Model file for the job. Use its own axes, mm. Face numbers are marked on the shaded views. Round coordinates to 2 decimals unless told otherwise and drop trailing zeros. Loops run counter-clockwise (first coordinate to the right, second up) from the corner with the lowest first, then second, coordinate; pieces in that order, holes last. Notation, with made-up numbers: M 41.5,39 L 57.5,39 A16 ccw 57.5,55 Z; hole C 89,83.5 d2. An arc over 180 degrees is marked long. Use a Markdown table: item, result. Add a question column.
Item 1: Saw through at C-C on x = -58. Write the cut outline in (y, z), then the cut area to 3 significant figures.
Item 2: Saw through at B-B on x = -4. Give the number of separate pieces and of enclosed holes in the cut face, then the cut area to 3 significant figures.
Item 3: Saw through at A-A on y = -32. Write the cut outline in (x, z), then the cut area to 3 significant figures.
Item 4: Pin check, flat tips, straight feed: P1, Ø8, axis at x = 56.5, y = 47, coming from the +Z side; P2, Ø3, axis at x = -75, z = 8.5, coming from the -Y side; P3, Ø3, axis at y = -90, z = 6, coming from the +X side. Stop position of each tip, or through.
Item 5: Two-plate mould, pull along X, no slides. Class the marked faces 1 and 2: +X half, -X half, draft (parallel to the pull), parting line (faces both ways), or undercut.
Item 6: Wall check: L1, parallel to Y at x = -74.3, z = 8; L2, parallel to Z at x = 71, y = 90; L3, parallel to X at y = -39.5, z = 9.5. Give the ranges that are in metal, low to high. Write a range as from..to.
```python
from build123d import *

# Parameters (mm, degrees)
SKETCH_W        = 153
SKETCH_H        = 228
SKETCH_R        = 1.75
PAD_DEPTH       = 3
SKETCH001_W     = 4
SKETCH001_H     = 190
PAD001_DEPTH    = 10
SKETCH002_R     = 1.75
POCKET_DEPTH    = 5
SKETCH003_R     = 1.15
POCKET001_DEPTH = 5


with BuildPart() as part:
    # Sketch → Pad (new body)
    with BuildSketch(Plane.XY):
        with Locations((0, 4)):
            Rectangle(SKETCH_W, SKETCH_H)
        with Locations((-23.5, 103)):
            Circle(SKETCH_R, mode=Mode.SUBTRACT)
        with Locations((-23.5, -103)):
            Circle(SKETCH_R, mode=Mode.SUBTRACT)
        with BuildLine():
            ThreePointArc((-50, 84.5), (-51.5, 83), (-50, 81.5))
            Line((-50, 81.5), (50, 81.5))
            ThreePointArc((50, 81.5), (51.5, 83), (50, 84.5))
            Line((-50, 84.5), (50, 84.5))
        make_face(mode=Mode.SUBTRACT)
        with BuildLine():
            ThreePointArc((-50, 77.5), (-51.5, 76), (-50, 74.5))
            Line((-50, 74.5), (50, 74.5))
            ThreePointArc((50, 74.5), (51.5, 76), (50, 77.5))
            Line((-50, 77.5), (50, 77.5))
        make_face(mode=Mode.SUBTRACT)
        with BuildLine():
            ThreePointArc((-50, 70.5), (-51.5, 69), (-50, 67.5))
            Line((-50, 67.5), (50, 67.5))
            ThreePointArc((50, 67.5), (51.5, 69), (50, 70.5))
            Line((-50, 70.5), (50, 70.5))
        make_face(mode=Mode.SUBTRACT)
        with BuildLine():
            ThreePointArc((-50, 63.5), (-51.5, 62), (-50, 60.5))
            Line((-50, 60.5), (50, 60.5))
            ThreePointArc((50, 60.5), (51.5, 62), (50, 63.5))
            Line((-50, 63.5), (50, 63.5))
        make_face(mode=Mode.SUBTRACT)
        with BuildLine():
            ThreePointArc((-50, 56.5), (-51.5, 55), (-50, 53.5))
            Line((-50, 53.5), (50, 53.5))
            ThreePointArc((50, 53.5), (51.5, 55), (50, 56.5))
            Line((-50, 56.5), (50, 56.5))
        make_face(mode=Mode.SUBTRACT)
        with BuildLine():
            ThreePointArc((-50, 49.5), (-51.5, 48), (-50, 46.5))
            Line((-50, 46.5), (50, 46.5))
            ThreePointArc((50, 46.5), (51.5, 48), (50, 49.5))
            Line((-50, 49.5), (50, 49.5))
        make_face(mode=Mode.SUBTRACT)
        with BuildLine():
            ThreePointArc((-50, 42.5), (-51.5, 41), (-50, 39.5))
            Line((-50, 39.5), (50, 39.5))
            ThreePointArc((50, 39.5), (51.5, 41), (50, 42.5))
            Line((-50, 42.5), (50, 42.5))
        make_face(mode=Mode.SUBTRACT)
        with BuildLine():
            ThreePointArc((-50, 35.5), (-51.5, 34), (-50, 32.5))
            Line((-50, 32.5), (50, 32.5))
            ThreePointArc((50, 32.5), (51.5, 34), (50, 35.5))
            Line((-50, 35.5), (50, 35.5))
        make_face(mode=Mode.SUBTRACT)
        with BuildLine():
            ThreePointArc((-50, 28.5), (-51.5, 27), (-50, 25.5))
            Line((-50, 25.5), (50, 25.5))
            ThreePointArc((50, 25.5), (51.5, 27), (50, 28.5))
            Line((-50, 28.5), (50, 28.5))
        make_face(mode=Mode.SUBTRACT)
        with BuildLine():
            ThreePointArc((-50, 21.5), (-51.5, 20), (-50, 18.5))
            Line((-50, 18.5), (50, 18.5))
            ThreePointArc((50, 18.5), (51.5, 20), (50, 21.5))
            Line((-50, 21.5), (50, 21.5))
        make_face(mode=Mode.SUBTRACT)
    extrude(amount=PAD_DEPTH)

    # Sketch001 → Pad001 (join)
    with BuildSketch(Plane.XY.offset(3)):
        with Locations((-74.5, 0)):
            Rectangle(SKETCH001_W, SKETCH001_H)
        with Locations((71.5, 0)):
            Rectangle(SKETCH001_W, SKETCH001_H)
    extrude(amount=PAD001_DEPTH)

    # Sketch002 → Pocket (cut)
    with BuildSketch(Plane.YZ.offset(-76.5)):
        with Locations((-85, 8)):
            Circle(SKETCH002_R)
        with Locations((0, 8)):
            Circle(SKETCH002_R)
        with Locations((85, 8)):
            Circle(SKETCH002_R)
    extrude(amount=POCKET_DEPTH, mode=Mode.SUBTRACT)

    # Sketch003 → Pocket001 (cut)
    with BuildSketch(Plane.YZ.offset(73.5)):
        with Locations((-90, 6)):
            Circle(SKETCH003_R)
        with Locations((0, 6)):
            Circle(SKETCH003_R)
        with Locations((90, 6)):
            Circle(SKETCH003_R)
    extrude(amount=-POCKET001_DEPTH, mode=Mode.SUBTRACT)


solid = part.part
```
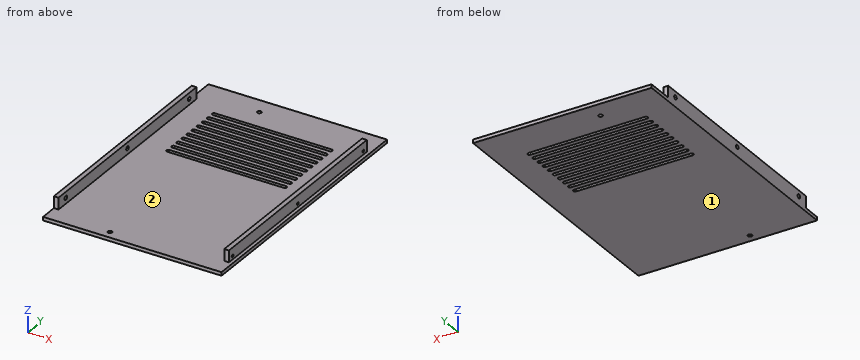
Entries:
| question | item | result |
|---|---|---|
| 1 | outline | M -110,0 L 118,0 L 118,3 L -110,3 Z |
| 1 | area | 684 mm2 |
| 2 | separate pieces | 11 |
| 2 | enclosed holes | 0 |
| 2 | area | 594 mm2 |
| 3 | outline | M -76.5,0 L 76.5,0 L 76.5,3 L 73.5,3 L 73.5,13 L 69.5,13 L 69.5,3 L -72.5,3 L -72.5,13 L -76.5,13 Z |
| 3 | area | 539 mm2 |
| 4 | P1 | z = 3 |
| 4 | P2 | y = -95 |
| 4 | P3 | x = 73.5 |
| 5 | face 1 | draft |
| 5 | face 2 | undercut |
| 6 | L1 | -95..-86.75, -83.25..-1.75, 1.75..83.25, 86.75..95 |
| 6 | L2 | 0..4.85, 7.15..13 |
| 6 | L3 | -76.5..-72.5, 69.5..73.5 |
